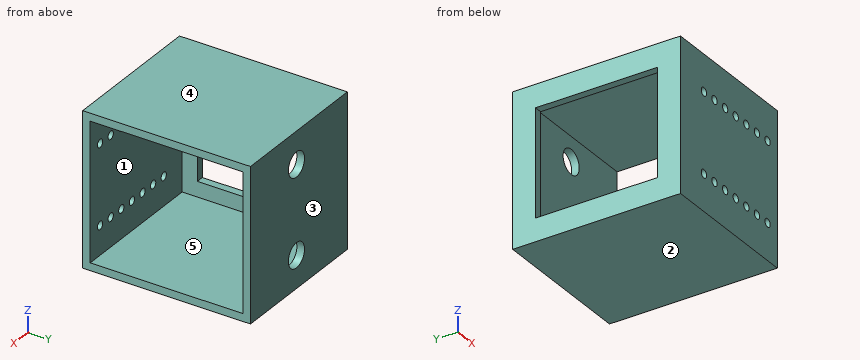
from build123d import *

# Parameters (mm, degrees)
BOSS_EXTRUDE1_DEPTH = 60
CUT_EXTRUDE1_REACH  = 104.255
SKETCH2_R           = 1.59
SKETCH3_W           = 42
SKETCH3_H           = 48
CUT_EXTRUDE2_DEPTH  = 60
SKETCH6_W           = 3
SKETCH6_H           = 60
BOSS_EXTRUDE2_DEPTH = 55
SKETCH4_R           = 4.826
CUT_EXTRUDE3_DEPTH  = 109.474


with BuildPart() as part:
    # Sketch1 → Boss-Extrude1 (new body)
    with BuildSketch(Plane.XY):
        Polygon((8, 30), (-47, 30), (-47, -30), (8, -30), (8, -33), (-50, -33), (-50, 33), (8, 33), align=None)
    extrude(amount=BOSS_EXTRUDE1_DEPTH)

    # Sketch2 → Cut-Extrude1 (cut, up to next)
    with BuildSketch(Plane.XZ.offset(33), mode=Mode.PRIVATE) as cut_extrude1_sk1:
        with Locations(Location((-36, 45.62, 0), (0, 0, 270))):
            Circle(SKETCH2_R)
    cut_extrude1_tool1 = extrude(cut_extrude1_sk1.sketch, amount=-CUT_EXTRUDE1_REACH, mode=Mode.PRIVATE) & part.part
    # Sketch2 → Cut-Extrude1 (cut, up to next)
    with BuildSketch(Plane.XZ.offset(33), mode=Mode.PRIVATE) as cut_extrude1_sk2:
        with Locations(Location((-29.65, 45.62, 0), (0, 0, 270))):
            Circle(SKETCH2_R)
    cut_extrude1_tool2 = extrude(cut_extrude1_sk2.sketch, amount=-CUT_EXTRUDE1_REACH, mode=Mode.PRIVATE) & part.part
    # Sketch2 → Cut-Extrude1 (cut, up to next)
    with BuildSketch(Plane.XZ.offset(33), mode=Mode.PRIVATE) as cut_extrude1_sk3:
        with Locations(Location((-23.3, 45.62, 0), (0, 0, 270))):
            Circle(SKETCH2_R)
    cut_extrude1_tool3 = extrude(cut_extrude1_sk3.sketch, amount=-CUT_EXTRUDE1_REACH, mode=Mode.PRIVATE) & part.part
    # Sketch2 → Cut-Extrude1 (cut, up to next)
    with BuildSketch(Plane.XZ.offset(33), mode=Mode.PRIVATE) as cut_extrude1_sk4:
        with Locations(Location((-16.95, 45.62, 0), (0, 0, 270))):
            Circle(SKETCH2_R)
    cut_extrude1_tool4 = extrude(cut_extrude1_sk4.sketch, amount=-CUT_EXTRUDE1_REACH, mode=Mode.PRIVATE) & part.part
    # Sketch2 → Cut-Extrude1 (cut, up to next)
    with BuildSketch(Plane.XZ.offset(33), mode=Mode.PRIVATE) as cut_extrude1_sk5:
        with Locations(Location((-10.6, 45.62, 0), (0, 0, 270))):
            Circle(SKETCH2_R)
    cut_extrude1_tool5 = extrude(cut_extrude1_sk5.sketch, amount=-CUT_EXTRUDE1_REACH, mode=Mode.PRIVATE) & part.part
    # Sketch2 → Cut-Extrude1 (cut, up to next)
    with BuildSketch(Plane.XZ.offset(33), mode=Mode.PRIVATE) as cut_extrude1_sk6:
        with Locations(Location((-4.25, 45.62, 0), (0, 0, 270))):
            Circle(SKETCH2_R)
    cut_extrude1_tool6 = extrude(cut_extrude1_sk6.sketch, amount=-CUT_EXTRUDE1_REACH, mode=Mode.PRIVATE) & part.part
    # Sketch2 → Cut-Extrude1 (cut, up to next)
    with BuildSketch(Plane.XZ.offset(33), mode=Mode.PRIVATE) as cut_extrude1_sk7:
        with Locations(Location((2.1, 45.62, 0), (0, 0, 270))):
            Circle(SKETCH2_R)
    cut_extrude1_tool7 = extrude(cut_extrude1_sk7.sketch, amount=-CUT_EXTRUDE1_REACH, mode=Mode.PRIVATE) & part.part
    # Sketch2 → Cut-Extrude1 (cut, up to next)
    with BuildSketch(Plane.XZ.offset(33), mode=Mode.PRIVATE) as cut_extrude1_sk8:
        with Locations(Location((-29.65, 14.38, 0), (0, 0, 270))):
            Circle(SKETCH2_R)
    cut_extrude1_tool8 = extrude(cut_extrude1_sk8.sketch, amount=-CUT_EXTRUDE1_REACH, mode=Mode.PRIVATE) & part.part
    # Sketch2 → Cut-Extrude1 (cut, up to next)
    with BuildSketch(Plane.XZ.offset(33), mode=Mode.PRIVATE) as cut_extrude1_sk9:
        with Locations(Location((-23.3, 14.38, 0), (0, 0, 270))):
            Circle(SKETCH2_R)
    cut_extrude1_tool9 = extrude(cut_extrude1_sk9.sketch, amount=-CUT_EXTRUDE1_REACH, mode=Mode.PRIVATE) & part.part
    # Sketch2 → Cut-Extrude1 (cut, up to next)
    with BuildSketch(Plane.XZ.offset(33), mode=Mode.PRIVATE) as cut_extrude1_sk10:
        with Locations(Location((-16.95, 14.38, 0), (0, 0, 270))):
            Circle(SKETCH2_R)
    cut_extrude1_tool10 = extrude(cut_extrude1_sk10.sketch, amount=-CUT_EXTRUDE1_REACH, mode=Mode.PRIVATE) & part.part
    # Sketch2 → Cut-Extrude1 (cut, up to next)
    with BuildSketch(Plane.XZ.offset(33), mode=Mode.PRIVATE) as cut_extrude1_sk11:
        with Locations(Location((-10.6, 14.38, 0), (0, 0, 270))):
            Circle(SKETCH2_R)
    cut_extrude1_tool11 = extrude(cut_extrude1_sk11.sketch, amount=-CUT_EXTRUDE1_REACH, mode=Mode.PRIVATE) & part.part
    # Sketch2 → Cut-Extrude1 (cut, up to next)
    with BuildSketch(Plane.XZ.offset(33), mode=Mode.PRIVATE) as cut_extrude1_sk12:
        with Locations(Location((-4.25, 14.38, 0), (0, 0, 270))):
            Circle(SKETCH2_R)
    cut_extrude1_tool12 = extrude(cut_extrude1_sk12.sketch, amount=-CUT_EXTRUDE1_REACH, mode=Mode.PRIVATE) & part.part
    # Sketch2 → Cut-Extrude1 (cut, up to next)
    with BuildSketch(Plane.XZ.offset(33), mode=Mode.PRIVATE) as cut_extrude1_sk13:
        with Locations(Location((2.1, 14.38, 0), (0, 0, 270))):
            Circle(SKETCH2_R)
    cut_extrude1_tool13 = extrude(cut_extrude1_sk13.sketch, amount=-CUT_EXTRUDE1_REACH, mode=Mode.PRIVATE) & part.part
    # Sketch2 → Cut-Extrude1 (cut, up to next)
    with BuildSketch(Plane.XZ.offset(33), mode=Mode.PRIVATE) as cut_extrude1_sk14:
        with Locations(Location((-36, 14.38, 0), (0, 0, 270))):
            Circle(SKETCH2_R)
    cut_extrude1_tool14 = extrude(cut_extrude1_sk14.sketch, amount=-CUT_EXTRUDE1_REACH, mode=Mode.PRIVATE) & part.part
    add(cut_extrude1_tool1.solids().sort_by_distance((-36, -33, 45.62))[0], mode=Mode.SUBTRACT)
    add(cut_extrude1_tool2.solids().sort_by_distance((-29.65, -33, 45.62))[0], mode=Mode.SUBTRACT)
    add(cut_extrude1_tool3.solids().sort_by_distance((-23.3, -33, 45.62))[0], mode=Mode.SUBTRACT)
    add(cut_extrude1_tool4.solids().sort_by_distance((-16.95, -33, 45.62))[0], mode=Mode.SUBTRACT)
    add(cut_extrude1_tool5.solids().sort_by_distance((-10.6, -33, 45.62))[0], mode=Mode.SUBTRACT)
    add(cut_extrude1_tool6.solids().sort_by_distance((-4.25, -33, 45.62))[0], mode=Mode.SUBTRACT)
    add(cut_extrude1_tool7.solids().sort_by_distance((2.1, -33, 45.62))[0], mode=Mode.SUBTRACT)
    add(cut_extrude1_tool8.solids().sort_by_distance((-29.65, -33, 14.38))[0], mode=Mode.SUBTRACT)
    add(cut_extrude1_tool9.solids().sort_by_distance((-23.3, -33, 14.38))[0], mode=Mode.SUBTRACT)
    add(cut_extrude1_tool10.solids().sort_by_distance((-16.95, -33, 14.38))[0], mode=Mode.SUBTRACT)
    add(cut_extrude1_tool11.solids().sort_by_distance((-10.6, -33, 14.38))[0], mode=Mode.SUBTRACT)
    add(cut_extrude1_tool12.solids().sort_by_distance((-4.25, -33, 14.38))[0], mode=Mode.SUBTRACT)
    add(cut_extrude1_tool13.solids().sort_by_distance((2.1, -33, 14.38))[0], mode=Mode.SUBTRACT)
    add(cut_extrude1_tool14.solids().sort_by_distance((-36, -33, 14.38))[0], mode=Mode.SUBTRACT)

    # Sketch3 → Cut-Extrude2 (cut)
    with BuildSketch(Plane.ZY.offset(50)):
        with Locations((30, 0)):
            Rectangle(SKETCH3_W, SKETCH3_H)
    extrude(amount=-CUT_EXTRUDE2_DEPTH, mode=Mode.SUBTRACT)

    # Sketch6 → Boss-Extrude2 (add)
    with BuildSketch(Plane(origin=(-47, 0, 0), x_dir=(0, 0, -1), z_dir=(1, 0, 0))):
        with Locations((-58.5, 0)):
            Rectangle(SKETCH6_W, SKETCH6_H)
        with Locations((-1.5, 0)):
            Rectangle(SKETCH6_W, SKETCH6_H)
    extrude(amount=BOSS_EXTRUDE2_DEPTH)

    # Sketch4 → Cut-Extrude3 (cut)
    with BuildSketch(Plane(origin=(-21.609229067, 30, -179.024422281), x_dir=(1, 0, 0), z_dir=(0, -1, 0))):
        with Locations((2.104243746, 226.324422281)):
            Circle(SKETCH4_R)
        with Locations((2.104243746, 191.724422281)):
            Circle(SKETCH4_R)
    extrude(amount=-CUT_EXTRUDE3_DEPTH, mode=Mode.SUBTRACT)


solid = part.part
Model file for the job. Use its own axes, mm. Face numbers are marked on the shaded views. A direction names the side the tool comes from. Give positions to 0.01 mm unless a question says otherwise; leave off trailing zeros. Write each loop counter-clockwise with the first axis right and the second up, starting at its lowest first coordinate (ties: lowest second). Pieces come first, ordered by that corner, then holes. Notation, with made-up numbers: (59, 76) - (76, 76) arc R25 cw to (76, 94) - close; hole circle Ø8 at (56.5, 18.5). An arc over 180 degrees is marked (long way). Answer as CSV lines item,"result".
1. Two-plate mould, pull along Y, no slides. Class the marked faces 1, 2 and 3: +Y half, -Y half, draft (parallel to the pull), parting line (faces both ways), or undercut.
Responses:
face 1,"undercut"
face 2,"draft"
face 3,"+Y half"
2. 3-axis set-ups, long thin cutter, end or side, ignore diameter. For the marked faces 4 and 5: which of +Z, -Z, +X, -X, +Y, -Y reach the whole face in a straight line?
Responses:
face 4,"+Z, +X, -X, +Y, -Y"
face 5,"+X"
3. Band-saw the part on A-A (y = -7.5). Write the cut outline in (x, z).
Responses:
outline,"(-50, 0) - (8, 0) - (8, 3) - (-47, 3) - (-47, 9) - (-50, 9) - close; (-50, 51) - (-47, 51) - (-47, 57) - (8, 57) - (8, 60) - (-50, 60) - close"
4. Drill centre lines: L1, parallel to Z at x = -28, y = -11; L2, parallel to Y at x = -34, z = 24; L3, parallel to Z at x = -10, y = -31. Where is each one in solid material? Low to high. Write a range as [from, to].
Responses:
L1,"z = [0, 3], [57, 60]"
L2,"y = [-33, -30], [30, 33]"
L3,"z = [0, 12.91], [15.85, 44.15], [47.09, 60]"
5. Band-saw the part on D-D (x = -23.3). Write the cut outline in (y, z), and give its area (3 significant figures).
Responses:
outline,"(-33, 0) - (33, 0) - (33, 9.72) - (30, 9.72) - (30, 3) - (-30, 3) - (-30, 12.79) - (-33, 12.79) - close; (-33, 15.97) - (-30, 15.97) - (-30, 44.03) - (-33, 44.03) - close; (-33, 47.21) - (-30, 47.21) - (-30, 57) - (30, 57) - (30, 50.28) - (33, 50.28) - (33, 60) - (-33, 60) - close; (30, 15.68) - (33, 15.68) - (33, 44.32) - (30, 44.32) - close"
area,"665 mm2"
6. Band-saw the part on C-C (z = 5). Write the cut outline in (x, y), and give its area (3 significant figures).
Responses:
outline,"(-50, -33) - (8, -33) - (8, -30) - (-47, -30) - (-47, 30) - (8, 30) - (8, 33) - (-50, 33) - close"
area,"528 mm2"
7. Band-saw the part on B-B (x = -36). Write the cut outline in (y, z), and give its area (3 significant figures).
Responses:
outline,"(-33, 0) - (33, 0) - (33, 60) - (-33, 60) - (-33, 47.21) - (-30, 47.21) - (-30, 57) - (30, 57) - (30, 3) - (-30, 3) - (-30, 12.79) - (-33, 12.79) - close; (-33, 15.97) - (-30, 15.97) - (-30, 44.03) - (-33, 44.03) - close"
area,"701 mm2"
8. Pin check, flat tips, straight feed: pin 1 (8 mm diameter, centred on x = -12.5, y = 4, fed in from -Z); pin 2 (1.9 mm diameter, centred on x = -36, z = 45.62, fed in from -Y). Stop position of each tip, or through.
Responses:
pin 1,"stops at z = 0"
pin 2,"stops at y = 30"
